Check sheet for the drawn part. Datum: minimum x, y, z corner. Units: mm. A direction names the side the tool comes from. Give positions to 0.01 mm unless a question says otherwise; leave off trailing zeros. Order: outer loops, then holes, each group sorted by start corner. A loop starts at its lowest first (then second) coordinate and runs counter-clockwise, first axis right, second up. Notation, with made-up numbers: (61.5, 70) -> (96.5, 70) arc R17 cw to (96.5, 75) -> close; hole circle Ø10 at (32.5, -2). An arc over 180 degrees is marked (long way). Answer in a Markdown table with one row per item. Add a question column.
(1) Cross-section at D-D (x = 38.5). Record the cut outline in (y, z).
(2) Cross-section at B-B (y = 1.45). Record the cut outline in (x, z).
(3) Thickness scan on L1, parallel to X at y = 0.75, z = 11.5; L2, parallel to X at y = 2.4, z = 11.5; L3, parallel to Z at x = 7, y = 1.1. Record the ranges inside material, lowest first. Write a range as [from, to].
(4) Cross-section at A-A (z = 11.5). Record the cut outline in (x, y).
(5) Go/stop test with flat-tipped pins: pin 1 (6 mm diameter, centred on x = 27, z = 10, fed in from +Y); pin 2 (4.5 mm diameter, centred on x = 32, z = 11.5, fed in from -Y). Record where each tip stops, or that it passes through.
(6) Cross-section at C-C (x = 32). Record the cut outline in (y, z), then the cut area to 3 significant figures.
(7) Release check for a two-part mould opening along X. For the marked faces 3, 4 and 5 record: released by +X, released by -X, zero draft, split by the parting line, or undercut.
(8) Set-up check for the marked faces 1 and 2: record each of +Z, -Z, +X, -X, +Y, -Y from which the full face is reachable in a straight line by a thin tool's end or side.
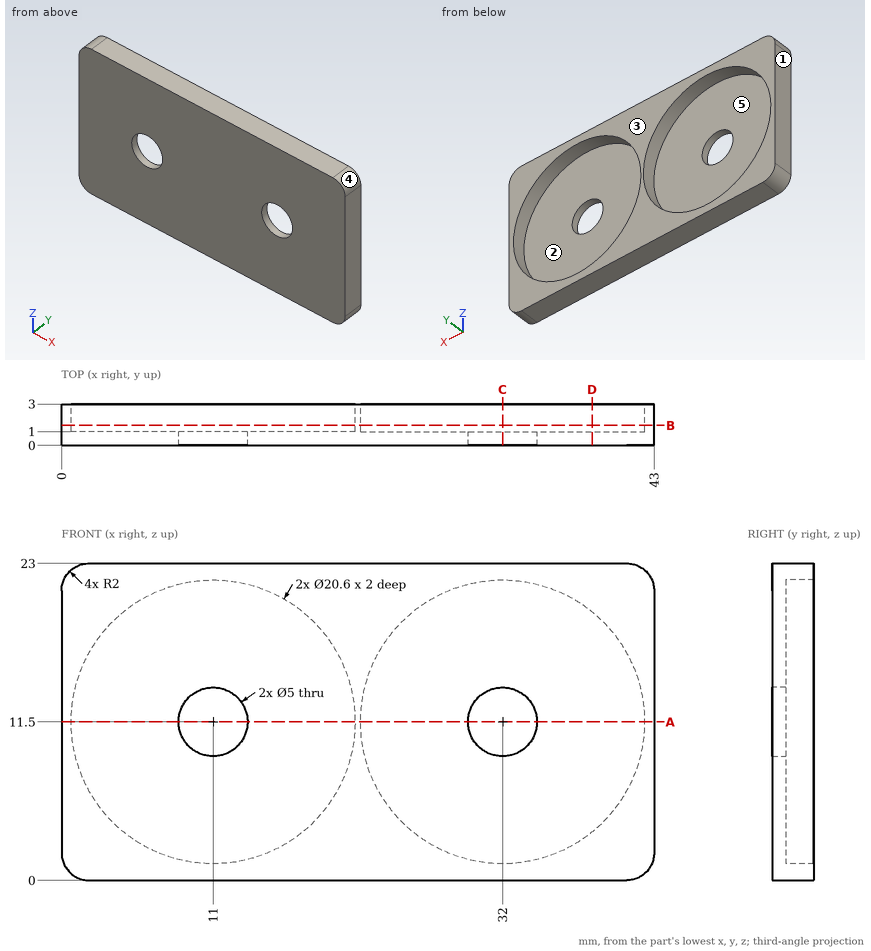
Answer below:
| question | item | result |
|---|---|---|
| 1 | outline | (0, 0) -> (3, 0) -> (3, 3.51) -> (1, 3.51) -> (1, 19.49) -> (3, 19.49) -> (3, 23) -> (0, 23) -> close |
| 2 | outline | (0, 2) arc R2 ccw to (2, 0) -> (41, 0) arc R2 ccw to (43, 2) -> (43, 21) arc R2 ccw to (41, 23) -> (2, 23) arc R2 ccw to (0, 21) -> close; hole circle Ø20.6 at (11, 11.5); hole circle Ø20.6 at (32, 11.5) |
| 3 | L1 | x = [0, 8.5], [13.5, 29.5], [34.5, 43] |
| 3 | L2 | x = [0, 0.7], [21.3, 21.7], [42.3, 43] |
| 3 | L3 | z = [0, 2.01], [20.99, 23] |
| 4 | outline | (0, 0) -> (8.5, 0) -> (8.5, 1) -> (0.7, 1) -> (0.7, 3) -> (0, 3) -> close; (13.5, 0) -> (29.5, 0) -> (29.5, 1) -> (21.7, 1) -> (21.7, 3) -> (21.3, 3) -> (21.3, 1) -> (13.5, 1) -> close; (34.5, 0) -> (43, 0) -> (43, 3) -> (42.3, 3) -> (42.3, 1) -> (34.5, 1) -> close |
| 5 | pin 1 | stops at y = 1 |
| 5 | pin 2 | passes through |
| 6 | outline | (0, 0) -> (3, 0) -> (3, 1.2) -> (1, 1.2) -> (1, 9) -> (0, 9) -> close; (0, 14) -> (1, 14) -> (1, 21.8) -> (3, 21.8) -> (3, 23) -> (0, 23) -> close |
| 6 | area | 22.8 mm² |
| 7 | face 3 | zero draft |
| 7 | face 4 | released by +X |
| 7 | face 5 | undercut |
| 8 | face 1 | +Z, -Z, -X, +Y, -Y |
| 8 | face 2 | +Y |
